```python
from build123d import *

# Parameters (mm, degrees)
SKETCH1_R           = 1.5
BOSS_EXTRUDE1_DEPTH = 5
CUT_EXTRUDE1_DEPTH  = 2.5
CUT_EXTRUDE3_DEPTH  = 1
SKETCH4_R           = 3
SKETCH4_R_2         = 1.5
EXTRUDE_THIN1_DEPTH = 1
CUT_EXTRUDE4_DEPTH  = 2
EXTRUDE_THIN2_REACH = 94.277
BOSS_EXTRUDE2_REACH = 94.277
FILLET1_R           = 3.5
BOSS_EXTRUDE8_DEPTH = 10


with BuildPart() as part:
    # Sketch1 → Boss-Extrude1 (new, symmetric)
    with BuildSketch(Plane.XY):
        with BuildLine():
            Line((0, 88.5), (-2, 86.5))
            Line((-2, 86.5), (0, 84.5))
            Line((0, 84.5), (-2, 82.5))
            Line((-2, 82.5), (0, 80.5))
            Line((0, 80.5), (-2, 78.5))
            Line((-2, 78.5), (0, 76.5))
            Line((0, 76.5), (0, 75))
            ThreePointArc((0, 75), (-5.309927761, 63.55), (0, 52.1))
            Line((0, 52.1), (-2, 50.1))
            Line((-2, 50.1), (0, 48.1))
            Line((0, 48.1), (-2, 46.1))
            Line((-2, 46.1), (0, 44.1))
            Line((0, 44.1), (-2, 42.1))
            ThreePointArc((-2, 42.1), (-4.035298286, 39.053960857), (-4.75, 35.460912703))
            Line((-4.75, 35.460912703), (-4.75, 0))
            ThreePointArc((-4.75, 0), (-11.25, -6.5), (-17.75, 0))
            Line((-17.75, 0), (-17.75, 67.916352203))
            Line((-17.75, 67.916352203), (-5, 90))
            Line((-5, 90), (0, 90))
            Line((0, 90), (0, 88.5))
        make_face()
        with Locations((-9.75, 0)):
            Circle(SKETCH1_R, mode=Mode.SUBTRACT)
        with Locations((-9.75, 25)):
            Circle(SKETCH1_R, mode=Mode.SUBTRACT)
    extrude(amount=BOSS_EXTRUDE1_DEPTH, both=True)

    # Sketch2 → Cut-Extrude1 (cut, symmetric)
    with BuildSketch(Plane.XY):
        with BuildLine():
            Line((-15, -8.410797367), (-15, 23.589202633))
            ThreePointArc((-15, 23.589202633), (-12.082951062, 31.431396204), (-4.75, 35.460912703))
            Line((-4.75, 35.460912703), (-4.75, -8.410797367))
            Line((-4.75, -8.410797367), (-15, -8.410797367))
        make_face()
    cut_extrude1 = extrude(amount=CUT_EXTRUDE1_DEPTH, both=True, mode=Mode.SUBTRACT)

    # Sketch3 → Cut-Extrude3 (cut)
    with BuildSketch(Plane.XY.offset(5)):
        with BuildLine():
            Line((-3.12764747, 88.5), (-4.133974596, 88.5))
            Line((-4.133974596, 88.5), (-16.25, 67.514428415))
            Line((-16.25, 67.514428415), (-16.25, 0))
            ThreePointArc((-16.25, 0), (-11.25, -5), (-6.25, 0))
            Line((-6.25, 0), (-6.25, 35.460912703))
            ThreePointArc((-6.25, 35.460912703), (-5.439227916, 39.583992212), (-3.12764747, 43.093084951))
            Line((-3.12764747, 43.093084951), (-3.12764747, 53.159809364))
            ThreePointArc((-3.12764747, 53.159809364), (-6.809927761, 63.55), (-3.12764747, 73.940190636))
            Line((-3.12764747, 73.940190636), (-3.12764747, 88.5))
        make_face()
    cut_extrude3 = extrude(amount=-CUT_EXTRUDE3_DEPTH, mode=Mode.SUBTRACT)

    # Sketch4 → Extrude-Thin1 (add)
    # profile 1 of 2: a face of its own
    with BuildSketch(Plane.XY.offset(4)):
        with Locations((-9.75, 25)):
            Circle(SKETCH4_R)
        with Locations((-9.75, 25)):
            Circle(SKETCH4_R_2, mode=Mode.SUBTRACT)
    # profile 2 of 2: a face of its own
    with BuildSketch(Plane.XY.offset(4)):
        with Locations((-9.75, 0)):
            Circle(SKETCH4_R)
        with Locations((-9.75, 0)):
            Circle(SKETCH4_R_2, mode=Mode.SUBTRACT)
    extrude_thin1 = extrude(amount=EXTRUDE_THIN1_DEPTH)

    # Sketch5 → Cut-Extrude4 (cut)
    with BuildSketch(Plane.XY.offset(4)):
        with BuildLine():
            Line((-16.25, 53.159809364), (-3.12764747, 53.159809364))
            ThreePointArc((-3.12764747, 53.159809364), (-6.809927761, 63.55), (-3.12764747, 73.940190636))
            Line((-3.12764747, 73.940190636), (-3.12764747, 88.5))
            Line((-3.12764747, 88.5), (-4.133974596, 88.5))
            Line((-4.133974596, 88.5), (-16.25, 67.514428415))
            Line((-16.25, 67.514428415), (-16.25, 53.159809364))
        make_face()
    cut_extrude4 = extrude(amount=-CUT_EXTRUDE4_DEPTH, mode=Mode.SUBTRACT)

    # Sketch6 → Extrude-Thin2 (add, up to next)
    with BuildSketch(Plane.XY.offset(5), mode=Mode.PRIVATE) as extrude_thin2_sk1:
        Polygon((-3.12764747, 54.159809364), (-13.401600212, 54.159809364), (-4.917118083, 60.954664271), (-14.27124031, 67.369931467), (-2.68786351, 73.042087041), (-3.56743143, 74.838294232), (-18.22875969, 67.658925362), (-8.271898443, 60.830286203), (-19.098399788, 52.159809364), (-3.12764747, 52.159809364), align=None)
    extrude_thin2_tool1 = extrude(extrude_thin2_sk1.sketch, amount=-EXTRUDE_THIN2_REACH, mode=Mode.PRIVATE) - part.part
    extrude_thin2 = extrude_thin2_tool1.solids().sort_by_distance((-8.264624, 53.879877, 5))[0]
    add(extrude_thin2)

    # Sketch7 → Boss-Extrude2 (add, up to next)
    with BuildSketch(Plane.XY.offset(5), mode=Mode.PRIVATE) as boss_extrude2_sk1:
        Polygon((-3.12764747, 73.940190636), (-3.56743143, 74.838294232), (-3.12764747, 75.053647931), align=None)
    boss_extrude2_tool1 = extrude(boss_extrude2_sk1.sketch, amount=-BOSS_EXTRUDE2_REACH, mode=Mode.PRIVATE) - part.part
    boss_extrude2 = boss_extrude2_tool1.solids().sort_by_distance((-3.274242, 74.610711, 5))[0]
    add(boss_extrude2)

    # Mirror2: Cut-Extrude1, Cut-Extrude3, Extrude-Thin1, Cut-Extrude4, Extrude-Thin2, Boss-Extrude2 across plane
    add(cut_extrude1.mirror(Plane.XY), mode=Mode.SUBTRACT)
    add(cut_extrude3.mirror(Plane.XY), mode=Mode.SUBTRACT)
    add(extrude_thin1.mirror(Plane.XY))
    add(cut_extrude4.mirror(Plane.XY), mode=Mode.SUBTRACT)
    add(extrude_thin2.mirror(Plane.XY))
    add(boss_extrude2.mirror(Plane.XY))

    # Fillet1
    fillet1_edges = [part.edges().sort_by_distance(p)[0] for p in [
        (-17.75, 67.916352203, 0),
        (-5, 90, 0),
    ]]
    fillet(fillet1_edges, radius=FILLET1_R)

    # Sketch11 → Boss-Extrude8 (add)
    with BuildSketch(Plane.XY.offset(5)):
        Polygon((0, 84.5), (0, 88.5), (-2, 86.5), align=None)
        Polygon((0, 80.5), (0, 84.5), (-2, 82.5), align=None)
        Polygon((0, 76.5), (0, 80.5), (-2, 78.5), align=None)
        Polygon((0, 48.1), (0, 52.1), (-2, 50.1), align=None)
        Polygon((0, 44.1), (0, 48.1), (-2, 46.1), align=None)
    extrude(amount=-BOSS_EXTRUDE8_DEPTH)


solid = part.part
```
Here's how the part is built. I have some questions about the finished solid (model axes, mm). A direction names the side the tool comes from. Give positions to 0.01 mm unless a question says otherwise; leave off trailing zeros. Loops run counter-clockwise (first coordinate to the right, second up) from the corner with the lowest first, then second, coordinate; pieces in that order, holes last. Notation, with made-up numbers: M 28.25,56.5 L 85.25,56.5 A19 ccw 85.25,84.5 Z; hole C 32.5,45.25 d5. An arc over 180 degrees is marked long. Return JSON: item names as keys, results as strings.
Item 1: I'm going to push flat-ended pins straight in: pin 1 Ø1.2 at (y, z) = (18.5, 3.5) entering from +X; pin 2 Ø1.5 at (y, z) = (5, 1) entering from +X; pin 3 Ø4 at (x, z) = (-11.5, 0) entering from -Y; pin 4 Ø2.5 at (x, y) = (-9.75, 25) entering from +Z. Where does each tip first touch, or does it pass through?
A:
{"pin 1": "stops at x = -4.75", "pin 2": "stops at x = -15", "pin 3": "stops at y = 29.4", "pin 4": "passes through"}
Item 2: On a 3-axis mill with a long thin cutter (end or side, diameter ignored), from which of +Z, -Z, +X, -X, +Y, -Y can I reach the whole of each face in a straight line? I mean faces 1 (the flat face through (-10.461, 64.757, 3.521)), 2 (the cylindrical face through (-12.131, 23.175, -4.493)), 3 (the cylindrical face through (-17.627, 67.897, 0.07)). Say none if no direction works.
A:
{"face 1": "+Z", "face 2": "-Z", "face 3": "+Z, -Z, -X, +Y"}
Item 3: Please list where these lines run through material, in increasing order: line 1 (X direction, y = 25, z = -3.2); line 2 (Y direction, x = -3.75, z = 3); line 3 (Z direction, x = -11.75, y = 4).
A:
{"line 1": "x = -17.75 to -11.25, -8.25 to -4.75", "line 2": "y = 39.68 to 56.89, 70.21 to 74.75, 88.5 to 89.91", "line 3": "z = -4 to -2.5, 2.5 to 4"}
Item 4: Imagine slicing it at C-C on y = 25. State how many separate pieces and enclosed holes the cut face has, then the cut area to 3 significant figures.
A:
{"separate pieces": "3", "enclosed holes": "0", "area": "56.2 mm^2"}
Item 5: Thinking about a two-plate mould opening in Y: for faces 4 (the cylindrical face through (-4.015, 39.102, 0.07)), 5 (the flat face through (-9, 54.16, 4)), 6 (the flat face through (-2, 90, 0)), which applies, released by +Y, released by -Y, zero draft, split by the parting line, or undercut?
A:
{"face 4": "released by -Y", "face 5": "undercut", "face 6": "released by +Y"}
Item 6: Imagine slicing it at B-B on z = 0.75. List the corners of the cut face in (x, y) for me, then the cut area to 3 significant figures.
A:
{"outline": "M -17.75,0 A6.5 ccw -15,-5.31 L -15,23.59 A12 cw -4.75,35.46 A9.39 cw -2,42.1 L 0,44.1 L 0,52.1 A15 cw 0,75 L 0,90 L -2.98,90 A3.5 ccw -6.01,88.25 L -17.28,68.73 A3.5 ccw -17.75,66.98 Z", "area": "852 mm^2"}
Item 7: Imagine slicing it at A-A on y = 45. List the corners of the cut face in (x, z) for me.
A:
{"outline": "M -17.75,-5 L -16.25,-5 L -16.25,-4 L -3.13,-4 L -3.13,-5 L 0,-5 L 0,5 L -3.13,5 L -3.13,4 L -16.25,4 L -16.25,5 L -17.75,5 Z"}
